Autodesk Inventor part; units mm, degrees
ref_plane "YZ Plane" through (0, 0, 0) normal (1, 0, 0) x (0, 1, 0)
ref_plane "XZ Plane" through (0, 0, 0) normal (0, 1, 0) x (-1, 0, 0)
ref_plane "XY Plane" through (0, 0, 0) normal (0, 0, 1) x (1, 0, 0)
sketch "Sketch1" plane through (0, 0, 0) normal (1, 0, 0) x (0, 1, 0)
  point P0 (0, 0)
sketch "Sketch2" plane through (0, 0, 0) normal (1, 0, 0) x (0, 1, 0)
  arc A0 (7.8808, -29.55) -> (0, -15.9) centre (0, -25) ccw
  arc A1 (9.9593, -30.75) -> (6.5, -15.5132) centre (0, -25) ccw
  line L0 (0, 0) -> (12.5, 0)
  line L1 (12.5, 0) -> (12.5, -4.5)
  line L2 (12.5, -4.5) -> (6.5, -4.5)
  line L3 (6.5, -4.5) -> (6.5, -15.5132)
  line L4 (7.8808, -29.55) -> (9.9593, -30.75)
  line L5 (0, -15.9) -> (0, 0)
  dimension "d0" = 4.5
  dimension "d2" = 18.2
  dimension "d3" = 23
  dimension "d5" = 25
  dimension "d7" = 12.5
  dimension "d8" = 6.5
  dimension "d9" = 60
revolve "Revolution1" add sketch "Sketch2" angle 360 about axis through (0, 0, -15.9) along (0, 0, 1)
hole "Hole1" at (0, 0, 0) direction (0, 0, -1) diameter 3 end through all
ref_plane "Work Plane1" through (0, 0, -16.2) normal (0, 0, -1) x (-1, 0, 0)
sketch "Sketch3" plane through (0, 0, -16.2) normal (0, 0, -1) x (-1, 0, 0)
  circle A0 centre (0, 0) radius 2.3668
hole "Hole2" at (0, 0, -16.2) direction (0, 0, 1) diameter 4.7336 depth 1.5
chamfer "Chamfer1" distance 0.5 angle 45 1 edges at (0, -12.5, 0)
chamfer "Chamfer2" distance 0.5 angle 45 1 edges at (0, -12.5, -4.5)
fillet "Fillet1" radius 5 1 edges at (0, -6.5, -4.5)
fillet "Fillet2" radius 3 1 edges at (0, -6.5, -15.5132)
sketch "Sketch4" plane through (0, 0, 0) normal (0, 0, 1) x (1, 0, 0)
  line L0 (4.5, -3.5) -> (4.5, 3.5)
  line L1 (4.5, 3.5) -> (6.5, 3.5)
  line L2 (6.5, 3.5) -> (6.5, -3.5)
  line L3 (6.5, -3.5) -> (4.5, -3.5)
  line L4 (-4.5, -3.5) -> (-6.5, -3.5)
  line L5 (-6.5, -3.5) -> (-6.5, 3.5)
  line L6 (-6.5, 3.5) -> (-4.5, 3.5)
  line L7 (-4.5, 3.5) -> (-4.5, -3.5)
  line L8 (0, 0) -> (0, -2.6483) construction
  line L9 (4.5, 0) -> (0, 0) construction
  dimension "d36" = 7
  dimension "d37" = 2
  dimension "d38" = 4.5
extrude "Extrusion1" add sketch "Sketch4" along normal blind 3
properties part number "vertebro_back"
Geometry: final body of the model. Coordinates: model frame, mm. A direction names the side the tool comes from. Give positions to 0.01 mm unless a question says otherwise; leave off trailing zeros. Write each loop counter-clockwise with the first axis right and the second up, starting at its lowest first coordinate (ties: lowest second). Pieces come first, ordered by that corner, then holes.
(1) Ray query, line 1 (Y direction, x = 0, z = -10.5); line 2 (X direction, y = 0, z = -3); line 3 (Z direction, x = 4, y = -6.25). Return the intervals inside material, ascending.
(2) Cut plane A-A, the plane z = -3. Return loops of the section in (x, y).
(3) Access query for faces 1 (the flat face through (5, 3.5, 1)), 2 (the flat face through (-6.5, 0, 1)), 3 (the cylindrical face through (-1.6, -1.744, -15.439)). Directions: +Z, -Z, +X, -X, +Y, -Y. A direction counts if a zero-diameter tool reaches every point of the face in a straight line with its end or side. Return the directions, or none.
(4) First-contact query: P1, Ø12, axis at x = -0.5, y = -1, coming from the -Z side; P2, Ø10, axis at y = 0, z = -20, coming from the -X side; P3, Ø7, axis at x = 1.5, y = 5, coming from the -Z side. Flat tips, straight axial feed; report the tip coordinate or a pass-through.
(5) Cut plane B-B, the plane z = -9. Return loops of the section in (x, y), then the cut area to 3 significant figures.
(6) Mould query, pull axis X, two halves, no side actions, for faces 4 (the flat face through (10, 6, -4.5)), 5 (the flat face through (-4.5, 0, 1)), 6 (the cylindrical face through (-3.955, -5.158, -11.805)). Classes: released by +X, released by -X, zero draft, split by the parting line, or undercut.
Values follow:
1. line 1: y = -6.5 to -1.5, 1.5 to 6.5
1. line 2: x = -12.5 to -1.5, 1.5 to 12.5
1. line 3: z = -19.73 to -16.21, -6.61 to 0
2. outline: circle Ø25 at (0, 0); hole circle Ø3 at (0, 0)
3. face 1: +Z, +X, -X, +Y
3. face 2: +Z, -X, +Y, -Y
3. face 3: none
4. P1: stops at z = -19.33
4. P2: stops at x = -11.5
4. P3: stops at z = -30.03
5. outline: circle Ø13.05 at (0, 0); hole circle Ø3 at (0, 0)
5. area: 127 mm2
6. face 4: zero draft
6. face 5: undercut
6. face 6: split by the parting line
